Autodesk Inventor part; units mm, degrees
ref_plane "YZ Plane" through (0, 0, 0) normal (1, 0, 0) x (0, 1, 0)
ref_plane "XZ Plane" through (0, 0, 0) normal (0, 1, 0) x (-1, 0, 0)
ref_plane "XY Plane" through (0, 0, 0) normal (0, 0, 1) x (1, 0, 0)
sketch "Эскиз1" plane through (0, 0, 0) normal (0, 1, 0) x (-1, 0, 0)
  line L0 (-51.75, 17.25) -> (51.75, 17.25)
  line L1 (51.75, 17.25) -> (51.75, -17.25)
  line L2 (51.75, -17.25) -> (-51.75, -17.25)
  line L3 (-51.75, -17.25) -> (-51.75, 17.25)
  line L4 (-51.75, 17.25) -> (51.75, -17.25) construction
  line L5 (51.75, 17.25) -> (-51.75, -17.25) construction
  line L6 (-41.75, -15.25) -> (0, -15.25)
  line L7 (41.75, -15.25) -> (41.75, -2.1292)
  line L8 (41.75, 15.25) -> (5.8292, 15.25)
  line L9 (-41.75, 15.25) -> (-41.75, -15.25)
  line L10 (0, -24.15) -> (0, 24.15) construction
  line L11 (0, -17.25) -> (0, -15.25) construction
  line L12 (0, 15.25) -> (0, 17.25) construction
  line L13 (0, -15.25) -> (41.75, 0)
  line L14 (41.75, 0) -> (0, 15.25)
  line L15 (5.8292, 15.25) -> (41.75, 2.1292)
  line L16 (41.75, -2.1292) -> (5.8292, -15.25)
  line L17 (41.75, -2.1292) -> (41.75, 2.1292) construction
  line L18 (41.75, 2.1292) -> (41.75, 15.25)
  line L19 (5.8292, -15.25) -> (41.75, -15.25)
  line L20 (0, -15.25) -> (5.8292, -15.25) construction
  line L21 (5.8292, 15.25) -> (0, 15.25) construction
  line L22 (0, 15.25) -> (-41.75, 15.25)
  line L23 (41.75, -2.1292) -> (41.0638, -0.2506) construction
  line L24 (41.75, 2.1292) -> (41.0638, 0.2506) construction
  point P0 (0, 0)
  point P1 (0, 0)
  dimension "d0" = 103.5
  dimension "d4" = 10
  dimension "d5" = 10
  dimension "d24" = 30.5
  dimension "d28" = 2
extrude "Выдавливание1" add sketch "Эскиз1" along normal blind 2
sketch "Эскиз2" plane through (0, 0, 0) normal (0, 1, 0) x (-1, 0, 0)
  line L0 (-41.75, -17.25) -> (-41.75, 17.25)
  line L1 (51.75, 17.25) -> (-51.75, 17.25)
  line L2 (-51.75, 17.25) -> (-51.75, -17.25)
  line L3 (0, -15.25) -> (-41.75, -15.25) construction
  line L4 (-39.75, -15.25) -> (-39.75, 15.25) construction
  line L5 (5.8292, 15.25) -> (41.75, 15.25) construction
  line L6 (-39.75, -15.25) -> (-24.5, -15.25) construction
  line L7 (-3.75, -15.25) -> (-3.75, -17.25)
  line L8 (-51.75, -17.25) -> (51.75, -17.25)
  line L9 (-3.75, -17.25) -> (-41.75, -17.25)
  line L10 (-41.75, 17.25) -> (-3.75, 17.25)
  line L11 (-3.75, 15.25) -> (-24.5, 15.25)
  line L12 (-3.75, 15.25) -> (-3.75, 17.25)
  arc A0 (-24.5, 15.25) -> (-24.5, -15.25) centre (-24.5, 0) ccw
  line L13 (-24.5, -15.25) -> (-3.75, -15.25)
  line L14 (-24.5, 15.25) -> (-39.75, 15.25) construction
  line L15 (-41.75, -15.25) -> (-41.75, 15.25)
  point P0 (0, 0)
  point P1 (41.75, -15.25)
  dimension "d13" = 2
  dimension "d14" = 36
extrude "Выдавливание2" add sketch "Эскиз2" along normal blind 13 contours L0 L1 L12 L11 A0 L13 L7 L8
sketch "Эскиз3" plane through (0, 2, 0) normal (0, 1, 0) x (1, 0, 0)
  line L0 (-41.75, 15.25) -> (-51.75, 15.25)
  line L1 (-51.75, 15.25) -> (-51.75, 17.25)
  line L2 (-51.75, 17.25) -> (-41.75, 17.25)
  line L3 (-41.75, 17.25) -> (-41.75, 15.25)
  line L4 (-51.75, 17.25) -> (-51.75, -17.25) construction
  line L5 (-51.75, -17.25) -> (-41.75, -17.25)
  line L6 (-41.75, -17.25) -> (-41.75, -15.25)
  line L7 (-41.75, -15.25) -> (-51.75, -15.25)
  line L8 (-51.75, -15.25) -> (-51.75, -17.25)
  point P0 (0, 0)
  point P1 (3.75, -15.25)
extrude "Выдавливание3" add sketch "Эскиз3" along normal blind 30
sketch "Эскиз5" plane through (0, 2, 0) normal (0, 1, 0) x (1, 0, 0)
  line L0 (51.75, 17.25) -> (51.75, -17.25) construction
  line L1 (51.75, -17.25) -> (41.75, -17.25) construction
  line L2 (41.75, 17.25) -> (41.75, -17.25) construction
  line L3 (3.75, 17.25) -> (41.75, 17.25) construction
  line L4 (3.75, 15.25) -> (3.75, 17.25) construction
  line L5 (3.75, 15.25) -> (0, 15.25) construction
  line L6 (0, 15.25) -> (-41.75, 0) construction
  line L7 (-41.75, 0) -> (0, -15.25) construction
  line L8 (0, -15.25) -> (3.75, -15.25) construction
  line L9 (3.75, -15.25) -> (24.5, -15.25) construction
  arc A0 (24.5, -15.25) -> (24.5, 15.25) centre (24.5, 0) ccw construction
  line L10 (24.5, 15.25) -> (3.75, 15.25) construction
  line L11 (41.75, 17.25) -> (51.75, 17.25) construction
  line L12 (41.75, -17.25) -> (3.75, -17.25) construction
  line L13 (3.75, -17.25) -> (3.75, -15.25) construction
  line L14 (-41.75, 17.25) -> (3.75, 17.25) construction
  line L15 (-41.75, 17.25) -> (-41.75, 15.25) construction
  line L16 (-5.8292, 15.25) -> (-41.75, 15.25) construction
  line L17 (-41.75, 2.1292) -> (-5.8292, 15.25) construction
  line L18 (-41.75, 15.25) -> (-41.75, 2.1292) construction
  line L19 (-41.75, 15.25) -> (-51.75, 15.25) construction
  line L20 (-51.75, 15.25) -> (-51.75, 17.25) construction
  line L21 (-51.75, 17.25) -> (-41.75, 17.25) construction
  line L22 (3.75, -17.25) -> (-41.75, -17.25) construction
  line L23 (-41.75, -15.25) -> (-41.75, -17.25) construction
  line L24 (-51.75, -15.25) -> (-41.75, -15.25) construction
  line L25 (-51.75, -17.25) -> (-51.75, -15.25) construction
  line L26 (-41.75, -17.25) -> (-51.75, -17.25) construction
  line L27 (-51.75, -15.25) -> (-51.75, 15.25) construction
  line L28 (-41.75, -15.25) -> (-5.8292, -15.25) construction
  line L29 (-5.8292, -15.25) -> (-41.75, -2.1292) construction
  line L30 (-41.75, -2.1292) -> (-41.75, -15.25) construction
  line L31 (-51.75, 17.25) -> (-41.75, -17.25) construction
  line L32 (-41.75, 17.25) -> (-51.75, -17.25) construction
  line L33 (51.75, 17.25) -> (-51.75, 17.25) construction
  line L34 (51.75, 17.25) -> (41.75, 0) construction
  line L35 (41.75, 17.25) -> (51.75, 0) construction
  line L36 (51.75, -17.25) -> (51.75, 17.25) construction
  line L37 (51.75, -17.25) -> (41.75, 0) construction
  line L38 (41.75, -17.25) -> (51.75, 0) construction
  circle A1 centre (-46.75, 0) radius 0.5
  circle A2 centre (46.75, 8.625) radius 0.5
  circle A3 centre (46.75, -8.625) radius 0.5
  point P0 (0, 0)
  dimension "d29" = 1
hole "Отверстие1" at (-46.75, 2, 0) at (46.75, 2, 8.625) at (46.75, 2, -8.625) direction (0, -1, 0) diameter 1 end through all countersink diameter 1.5 countersink angle 90
sketch "Эскиз4" plane through (-51.75, 0, 17.25) normal (0, 0, 1) x (1, 0, 0)
  line L0 (10, 32) -> (0, 32) construction
  line L1 (0, 32) -> (10, 32) construction
  line L2 (10, 32) -> (10, 22) construction
  line L3 (10, 22) -> (0, 22) construction
  line L4 (0, 22) -> (0, 32) construction
  line L5 (103.5, 0) -> (0, 0) construction
  line L6 (0, 0) -> (0, 32) construction
  line L7 (10, 32) -> (10, 2) construction
  line L8 (10, 2) -> (55.5, 2) construction
  line L9 (55.5, 2) -> (55.5, 13) construction
  line L10 (55.5, 13) -> (93.5, 13) construction
  line L11 (93.5, 13) -> (93.5, 2) construction
  line L12 (93.5, 2) -> (103.5, 2) construction
  line L13 (103.5, 2) -> (103.5, 0) construction
  line L14 (10, 2) -> (10, 32) construction
  line L15 (0, 0) -> (0, 32) construction
  line L16 (10, 22) -> (0, 32) construction
  line L17 (10, 32) -> (0, 22) construction
  circle A0 centre (5, 27) radius 0.5
  line L18 (55.5, 13) -> (65.5, 13) construction
  line L19 (65.5, 13) -> (65.5, 3) construction
  line L20 (65.5, 3) -> (55.5, 3) construction
  line L21 (55.5, 3) -> (55.5, 13) construction
  line L22 (65.5, 13) -> (55.5, 3) construction
  line L23 (55.5, 2) -> (55.5, 13) construction
  line L24 (55.5, 13) -> (65.5, 3) construction
  circle A1 centre (60.5, 8) radius 0.5
  line L25 (0, 32) -> (10, 32)
  point P0 (51.75, 0)
  dimension "d19" = 1
  dimension "d20" = 10
  dimension "d21" = 1
hole "Отверстие2" at (-46.75, 27, 17.25) at (8.75, 8, 17.25) direction (0, 0, -1) diameter 1 depth 17.25 countersink diameter 1.5 countersink angle 90
mirror "Зеркальное отражение1" about plane through (0, 0, 0) normal (0, 0, 1) of "Отверстие2"
properties part number "frame"
Build history of the part. All positions in model axes, mm. A direction names the side the tool comes from. Give positions to 0.01 mm unless a question says otherwise; leave off trailing zeros. Loops run counter-clockwise (first coordinate to the right, second up) from the corner with the lowest first, then second, coordinate; pieces in that order, holes last.
1) Two-plate mould, pull along Z, no slides. Class faces 4 (the face through (-4.1, 1.7, -17.25)), 5 (the face through (-21.167, 0.986, 7.518)), 6 (the face through (-41.75, 17, 16)), 7 (the face through (-36, 2, 4)): released by +Z, released by -Z, zero draft, split by the parting line, or undercut.
Values follow:
face 4: released by -Z
face 5: undercut
face 6: zero draft
face 7: undercut
2) Drop flat-ended pins along their axis: P1, Ø3, axis at x = 46.5, z = 4.5, coming from the +Y side; P2, Ø10, axis at y = 7.5, z = 3.5, coming from the +X side; P3, Ø4, axis at y = 8.5, z = 0, coming from the -X side; P4, Ø17, axis at x = 19.5, z = 1.5, coming from the +Y side. Give the stop position or say it passes through.
Values follow:
P1: stops at y = 2
P2: stops at x = 41.75
P3: stops at x = 39.62
P4: passes through
3) Band-saw the part on A-A on y = 21.5. List the corners of the cut face in (x, z), then the cut area to 3 significant figures.
Values follow:
outline: (-51.75, -17.25) - (-41.75, -17.25) - (-41.75, -15.25) - (-51.75, -15.25) - close; (-51.75, 15.25) - (-41.75, 15.25) - (-41.75, 17.25) - (-51.75, 17.25) - close
area: 40.0 mm2
4) Probe line 1 along X through (y, z) = (8, -16); line 2 along Z through (x, y) = (16, 7); line 3 along Z through (x, y) = (-24, 1). List the from-to ranges inside material, lowest first.
Values follow:
line 1: x = -51.75 to -41.75, 3.75 to 8.25, 9.25 to 41.75
line 2: z = -17.25 to -15.25, 15.25 to 17.25
line 3: z = -17.25 to -15.25, -8.61 to -6.48, 6.48 to 8.61, 15.25 to 17.25
5) 3-axis set-ups, long thin cutter, end or side, ignore diameter. For faces 1 (the face through (-20.583, 0.986, -7.732)), 2 (the face through (-47, 17, 15.25)), 3 (the face through (40, 13, 1)): which of +Z, -Z, +X, -X, +Y, -Y reach the whole face in a straight line?
Values follow:
face 1: +Y, -Y
face 2: -X, +Y
face 3: +Z, -Z, +X, +Y
6) Band-saw the part on C-C on z = -12. List the corners of the cut face in (x, y).
Values follow:
outline: (-51.75, 0) - (-41.75, 0) - (-41.75, 2) - (-51.75, 2) - close; (-14.73, 0) - (-8.9, 0) - (-8.9, 2) - (-14.73, 2) - close; (33.91, 0) - (51.75, 0) - (51.75, 2) - (41.75, 2) - (41.75, 13) - (33.91, 13) - close
7) Band-saw the part on D-D on z = 4.5. List the corners of the cut face in (x, y).
Values follow:
outline: (-51.75, 0) - (-41.75, 0) - (-41.75, 2) - (-51.75, 2) - close; (-35.26, 0) - (-29.43, 0) - (-29.43, 2) - (-35.26, 2) - close; (39.07, 0) - (51.75, 0) - (51.75, 2) - (41.75, 2) - (41.75, 13) - (39.07, 13) - close
8) Band-saw the part on B-B on x = 14.5. List the corners of the cut face in (y, z).
Values follow:
outline: (0, -17.25) - (13, -17.25) - (13, -15.25) - (0, -15.25) - close; (0, 15.25) - (13, 15.25) - (13, 17.25) - (0, 17.25) - close
